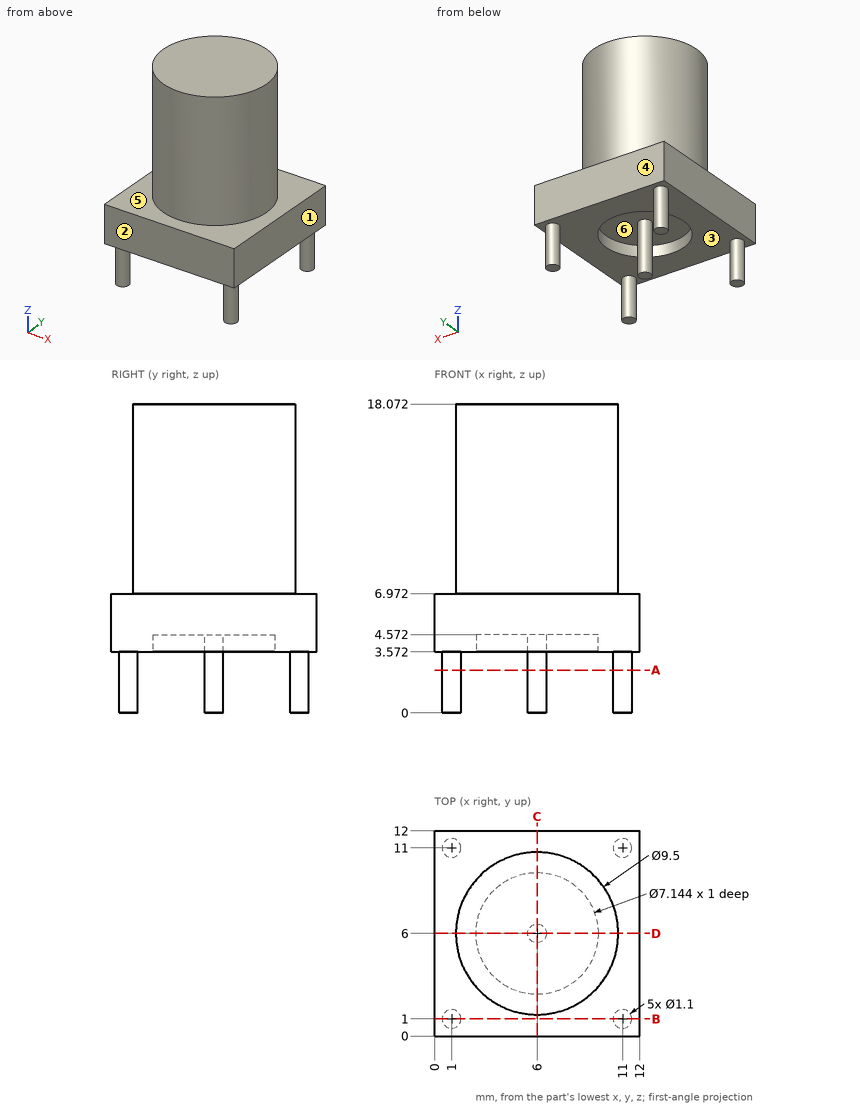
Source: three-view drawing plus pictorial views. Frame: mm from the lowest corner of the part. A direction names the side the tool comes from. Round coordinates to 2 decimals unless told otherwise and drop trailing zeros. Write each loop counter-clockwise with the first axis right and the second up, starting at its lowest first coordinate (ties: lowest second). Pieces come first, ordered by that corner, then holes. Notation, with made-up numbers: M -26.5,-36.75 L 31.5,-36.75 A28 ccw 31.5,-0.75 Z; hole C 64,58.5 d3. An arc over 180 degrees is marked long. One line per item, written item: value. Start each with the question number.
Item 1: Section query B-B (y = 1). Return the cut outline in (x, z).
Item 2: Section query C-C (x = 6). Return the cut outline in (y, z), plus the area to 3 significant figures.
Item 3: Mould query, pull axis Y, two halves, no side actions, for the marked faces 1, 2 and 3. Classes: pulls with the +Y half, pulls with the -Y half, needs draft (parallel to the pull), parting line crosses it, or undercut.
Item 4: Ray query, L1, parallel to Y at x = 6, z = 3.9; L2, parallel to Z at x = 9, y = 5.25. Return the intervals inside material, ascending. Write a range as from..to.
Item 5: Pin query (flat end, axial travel): pin 1 (4 mm diameter, centred on y = 9.5, z = 7, fed in from +X); pin 2 (3 mm diameter, centred on x = 1.5, z = 14.5, fed in from -Y); pin 3 (1 mm diameter, centred on x = 4, y = 7.5, fed in from -Z); pin 4 (1.5 mm diameter, centred on y = 2, z = 10.5, fed in from +X). Return the tip coordinate at first contact, or that it passes through.
Item 6: Section query A-A (z = 2.5). Return the cut outline in (x, y).
Item 7: Set-up query: the marked faces 4, 5 and 6. Return all of +Z, -Z, +X, -X, +Y, -Y with unobstructed straight access to the full face (end or side cutting, diameter ignored); none if empty.
Result set:
1. outline: M 0,3.57 L 0.45,3.57 L 0.45,0 L 1.55,0 L 1.55,3.57 L 10.45,3.57 L 10.45,0 L 11.55,0 L 11.55,3.57 L 12,3.57 L 12,6.97 L 0,6.97 Z
2. outline: M 0,3.57 L 2.43,3.57 L 2.43,4.57 L 5.45,4.57 L 5.45,0 L 6.55,0 L 6.55,4.57 L 9.57,4.57 L 9.57,3.57 L 12,3.57 L 12,6.97 L 10.75,6.97 L 10.75,18.07 L 1.25,18.07 L 1.25,6.97 L 0,6.97 Z
2. area: 144 mm²
3. face 1: needs draft
3. face 2: pulls with the -Y half
3. face 3: undercut
4. L1: y = 0..2.43, 5.45..6.55, 9.57..12
4. L2: z = 4.57..18.07
5. pin 1: stops at x = 12
5. pin 2: stops at y = 2.32
5. pin 3: stops at z = 4.57
5. pin 4: stops at x = 9.46
6. outline: C 1,1 d1.1; C 1,11 d1.1; C 6,6 d1.1; C 11,1 d1.1; C 11,11 d1.1
7. face 4: +Z, -Z, +X, -X, +Y
7. face 5: +Z
7. face 6: -Z
